Source: three-view drawing plus pictorial views. Frame: mm from the lowest corner of the part. A direction names the side the tool comes from. Coordinates: 2 decimals unless noted, no trailing zeros. Write each loop counter-clockwise with the first axis right and the second up, starting at its lowest first coordinate (ties: lowest second). Pieces come first, ordered by that corner, then holes. Notation, with made-up numbers: (82.25, -29.5) -> (89.25, -29.5) arc R24 cw to (89.25, 8.5) -> close; hole circle Ø2 at (-17, -10). An arc over 180 degrees is marked (long way). One line per item, written item: value. Start each with the question number.
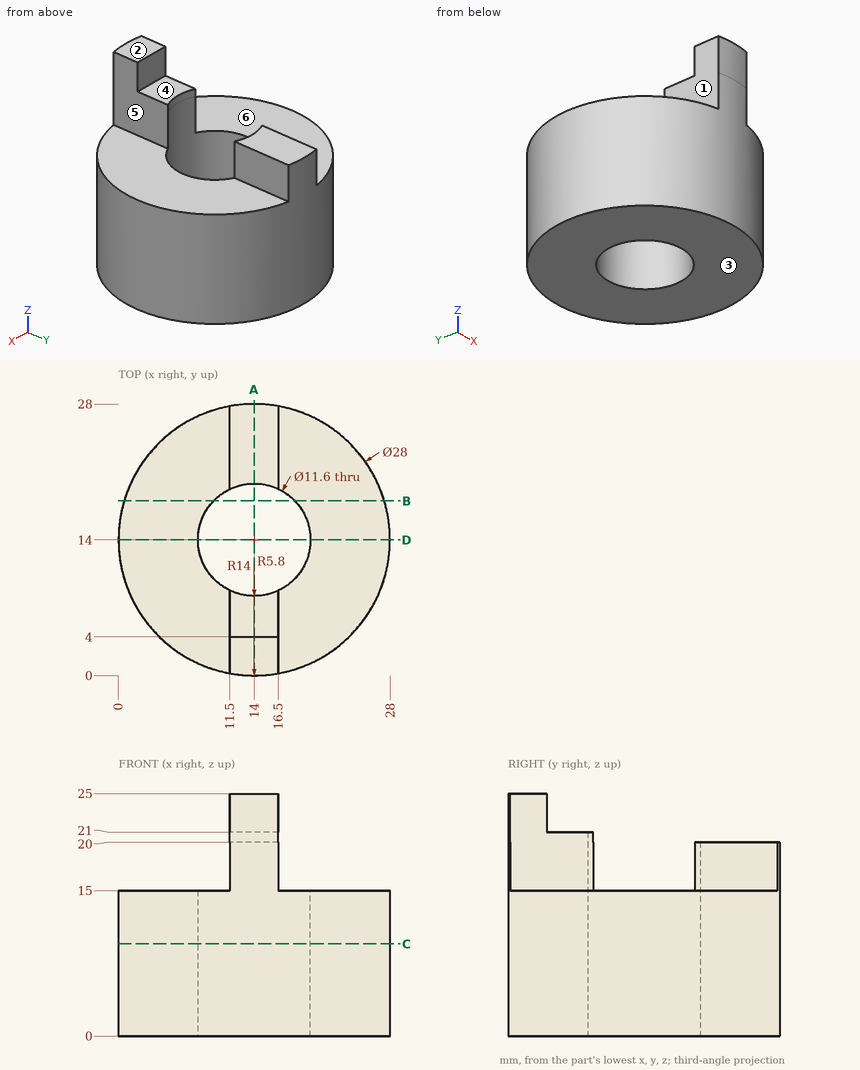
Q1. Access query for the marked faces 4, 5 and 6. Directions: +Z, -Z, +X, -X, +Y, -Y. A direction counts if a zero-diameter tool reaches every point of the face in a straight line with its end or side. Return the directions, or none.
Q2. First-contact query: P1, Ø9.5, axis at y = 6, z = 21.5, coming from the +X side; P2, Ø4, axis at y = 24, z = 18.5, coming from the -X side; P3, Ø9.5, axis at y = 4, z = 19.5, coming from the -X side. Flat tips, straight axial feed; report the tip coordinate or a pass-through.
Q3. Cut plane C-C on z = 9.5. Output: boundary loops of the cut face in (x, y).
Q4. Line query: L1, parallel to Y at x = 14.25, z = 10.75; L2, parallel to X at y = 14, z = 9.5; L3, parallel to Z at x = 15, y = 26. Output: solid intervals per line, ascending. Write a range as from..to.
Q5. Cut plane A-A on x = 14. Output: boundary loops of the cut face in (y, z).
Q6. Cut plane B-B on y = 18. Output: boundary loops of the cut face in (x, z), and give its area (3 significant figures).
Q7. Cut plane D-D on y = 14. Output: boundary loops of the cut face in (x, z), and give its area (3 significant figures).
Q8. Draft query along Z for the marked faces 1, 2 and 3. Return one class per face: pulls with the +Z half, pulls with the -Z half, needs draft (parallel to the pull), parting line crosses it, or undercut.
Solution:
1. face 4: +Z, +X, -X, +Y
1. face 5: +Z, +X, +Y, -Y
1. face 6: +Z, -X, +Y, -Y
2. P1: x = 16.5
2. P2: x = 11.5
2. P3: x = 2.86
3. outline: circle Ø28 at (14, 14); hole circle Ø11.6 at (14, 14)
4. L1: 0..8.21, 19.79..28
4. L2: 0..8.2, 19.8..28
4. L3: 0..20
5. outline: (0, 0) -> (8.2, 0) -> (8.2, 21) -> (4, 21) -> (4, 25) -> (0, 25) -> close; (19.8, 0) -> (28, 0) -> (28, 20) -> (19.8, 20) -> close
6. outline: (0.58, 0) -> (9.8, 0) -> (9.8, 15) -> (0.58, 15) -> close; (18.2, 0) -> (27.42, 0) -> (27.42, 15) -> (18.2, 15) -> close
6. area: 276 mm²
7. outline: (0, 0) -> (8.2, 0) -> (8.2, 15) -> (0, 15) -> close; (19.8, 0) -> (28, 0) -> (28, 15) -> (19.8, 15) -> close
7. area: 246 mm²
8. face 1: needs draft
8. face 2: pulls with the +Z half
8. face 3: pulls with the -Z half
